Autodesk Inventor part; units mm, degrees
ref_plane "YZ Plane" through (0, 0, 0) normal (1, 0, 0) x (0, 1, 0)
ref_plane "XZ Plane" through (0, 0, 0) normal (0, 1, 0) x (-1, 0, 0)
ref_plane "XY Plane" through (0, 0, 0) normal (0, 0, 1) x (1, 0, 0)
sketch "Sketch1" plane through (0, 0, 0) normal (0, 1, 0) x (-1, 0, 0)
  circle A0 centre (0, 0) radius 11.05
  line L0 (21.25, 17.25) -> (21.25, -17.25)
  line L1 (21.25, -17.25) -> (17.25, -21.25)
  line L2 (17.25, -21.25) -> (-17.25, -21.25)
  line L3 (-17.25, -21.25) -> (-21.25, -17.25)
  line L4 (-21.25, -17.25) -> (-21.25, 17.25)
  line L5 (-21.25, 17.25) -> (-17.25, 21.25)
  line L6 (-17.25, 21.25) -> (17.25, 21.25)
  line L7 (17.25, 21.25) -> (21.25, 17.25)
  line L8 (21.25, 0) -> (-21.25, 0) construction
  line L9 (0, 21.25) -> (0, -21.25) construction
  circle A1 centre (15.3506, -15.3506) radius 1.55
  line L10 (15.3506, -15.3506) -> (0, 0) construction
  circle A2 centre (15.3506, 15.3506) radius 1.55
  circle A3 centre (-15.3506, 15.3506) radius 1.55
  circle A4 centre (-15.3506, -15.3506) radius 1.55
  point P0 (0, 0)
  dimension "d0" = 22.1
  dimension "d1" = 135
  dimension "d2" = 42.5
  dimension "d3" = 5.6569
  dimension "d25" = 3.1
  dimension "d26" = 21.709
  dimension "d27" = 45
  dimension "d30" = 360
extrude "Extrusion1" add sketch "Sketch1" along normal blind 6
sketch "Sketch6" plane through (0, 0, 0) normal (0, -1, 0) x (1, 0, 0)
  line L0 (27.25, -23.25) -> (27.25, 23.25)
  line L1 (27.25, 23.25) -> (23.25, 27.25)
  line L2 (23.25, 27.25) -> (-23.25, 27.25)
  line L3 (-23.25, 27.25) -> (-27.25, 23.25)
  line L4 (-27.25, 23.25) -> (-27.25, -23.25)
  line L5 (-27.25, -23.25) -> (-23.25, -27.25)
  line L6 (-23.25, -27.25) -> (23.25, -27.25)
  line L7 (23.25, -27.25) -> (27.25, -23.25)
  line L8 (25.25, -25.25) -> (-25.25, 25.25) construction
  line L9 (-17.25, 21.25) -> (17.25, 21.25) construction
  line L10 (23.25, 27.25) -> (17.25, 21.25) construction
  line L11 (27.25, 23.25) -> (21.25, 17.25) construction
  line L12 (21.25, -17.25) -> (17.25, -21.25)
  line L13 (21.25, 17.25) -> (21.25, -17.25)
  line L14 (21.25, -17.25) -> (21.25, 17.25)
  line L15 (17.25, 21.25) -> (21.25, 17.25)
  line L16 (21.25, 17.25) -> (17.25, 21.25)
  line L17 (17.25, 21.25) -> (-17.25, 21.25)
  line L18 (-21.25, 17.25) -> (-17.25, 21.25)
  line L19 (-21.25, 17.25) -> (-17.25, 21.25)
  line L20 (17.25, 21.25) -> (21.25, 17.25)
  line L21 (-21.25, -17.25) -> (-21.25, 17.25)
  line L22 (-21.25, 17.25) -> (-21.25, -17.25)
  line L23 (-21.25, -17.25) -> (-17.25, -21.25)
  line L24 (-17.25, -21.25) -> (17.25, -21.25)
  line L25 (17.25, -21.25) -> (21.25, -17.25)
  point P0 (0, 0)
  point P1 (0, 0)
  dimension "d32" = 135
  dimension "d33" = 135
  dimension "d34" = 46.5
extrude "Extrusion5" add sketch "Sketch6" against normal blind 41
sketch "Sketch8" plane through (0, 41, 0) normal (0, 1, 0) x (1, 0, 0)
  line L0 (27.25, -23.25) -> (27.25, 23.25)
  line L1 (21.25, -17.25) -> (21.25, 17.25)
  line L2 (27.25, 23.25) -> (21.25, 17.25)
  line L3 (17.25, -21.25) -> (21.25, -17.25)
  line L4 (21.25, 17.25) -> (21.25, -17.25)
  line L5 (21.25, -17.25) -> (27.25, -23.25)
  line L6 (27.25, -23.25) -> (27.25, 23.25)
  point P0 (0, 0)
  point P1 (27.25, -23.25)
extrude "Extrusion6" cut sketch "Sketch8" against normal blind 35
sketch "Sketch9" plane through (0, 6, 0) normal (0, 1, 0) x (1, 0, 0)
  line L0 (23.25, 27.25) -> (-23.25, 27.25)
  line L1 (17.25, 21.25) -> (21.25, 17.25)
  line L2 (23.25, 27.25) -> (17.25, 21.25)
  line L3 (-21.25, 17.25) -> (-17.25, 21.25)
  line L4 (17.25, 21.25) -> (-17.25, 21.25)
  line L5 (-17.25, 21.25) -> (-23.25, 27.25)
  line L6 (-23.25, 27.25) -> (23.25, 27.25)
  line L7 (-17.25, -21.25) -> (17.25, -21.25)
  line L8 (23.25, -27.25) -> (-23.25, -27.25)
  line L9 (17.25, -21.25) -> (23.25, -27.25)
  line L10 (23.25, -27.25) -> (-23.25, -27.25)
  line L11 (-23.25, -27.25) -> (-17.25, -21.25)
  line L12 (-17.25, -21.25) -> (17.25, -21.25)
  point P0 (0, 0)
  point P1 (-23.25, 27.25)
extrude "Extrusion7" cut sketch "Sketch9" along normal blind 29
sketch "Sketch10" plane through (-21.25, 6, -17.25) normal (1, 0, 0) x (0, 0, -1)
  line L0 (6, 0) -> (-40.5, 0) construction
  line L1 (-17.25, 0) -> (-17.25, 35) construction
  line L2 (-34.5, 35) -> (0, 35) construction
  line L3 (0, 0) -> (0, 35) construction
  line L4 (0, 17.5) -> (-34.5, 17.5) construction
  line L5 (-34.5, 0) -> (-34.5, 35) construction
  line L6 (-32.5, 2) -> (-2, 2)
  line L7 (-2, 2) -> (-2, 33)
  line L8 (-2, 33) -> (-32.5, 33)
  line L9 (-32.5, 33) -> (-32.5, 2)
  line L10 (-17.25, 2) -> (-17.25, 33) construction
  line L11 (-32.5, 17.5) -> (-2, 17.5) construction
  point P0 (-17.25, -6)
  point P1 (-17.25, 17.5)
  dimension "d41" = 2
  dimension "d42" = 2
extrude "Extrusion8" cut sketch "Sketch10" against normal blind 2
sketch "Sketch11" plane through (-23.25, 6, -17.25) normal (1, 0, 0) x (0, 0, -1)
  line L0 (-7.2, 7.5) -> (-27.3, 7.5) construction
  line L1 (-27.3, 7.5) -> (-27.3, 27.5) construction
  line L2 (-27.3, 27.5) -> (-7.2, 27.5) construction
  line L3 (-7.2, 27.5) -> (-7.2, 7.5) construction
  line L4 (-2, 33) -> (-2, 2) construction
  line L5 (-32.5, 2) -> (-32.5, 33) construction
  line L6 (-2, 2) -> (-32.5, 33) construction
  line L7 (-32.5, 33) -> (-2, 33) construction
  line L8 (-32.5, 2) -> (-2, 33) construction
  line L9 (-7.2, 7.5) -> (-27.3, 27.5) construction
  line L10 (-27.3, 7.5) -> (-7.2, 27.5) construction
  point P0 (-17.25, -6)
  point P1 (-17.25, 17.5)
  dimension "d45" = 20.1
  dimension "d46" = 20
hole "Hole2" at (-23.25, 13.5, -10.05) at (-23.25, 13.5, 10.05) at (-23.25, 33.5, -10.05) at (-23.25, 33.5, 10.05) direction (-1, 0, 0) diameter 3 depth 4
equation "\"d0\" = shaft_hole_diameter"
equation "\"d4\" = mount_face_thickness"
equation "\"d34\" = mount_width"
equation "\"d35\" = mount_length"
equation "\"d37\" = mount_length - mount_face_thickness"
equation "\"d39\" = mount_length - 2 * mount_face_thickness"
equation "\"d45\" = screw_x"
equation "\"d46\" = screw_y"
equation "\"d47\" = screw_diameter"
equation "\"shaft_hole_diameter\" = 22.1"
equation "\"mount_width\" = 46.5"
equation "\"mount_slant_length\" = 5"
equation "\"mount_face_thickness\" = 6"
equation "\"mount_length\" = 41"
equation "\"screw_x\" = 20.1"
equation "\"screw_y\" = 20"
equation "\"screw_diameter\" = 3"
properties part number "table_motor_mount"
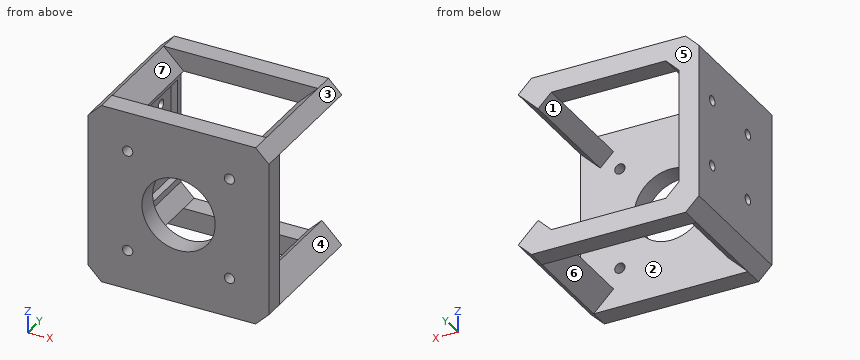
The model under review builds one solid part; all positions refer to its coordinate system, in mm. Face numbers are marked on the shaded views. A direction names the side the tool comes from. Round coordinates to 2 decimals unless told otherwise and drop trailing zeros. Loops run counter-clockwise (first coordinate to the right, second up) from the corner with the lowest first, then second, coordinate; pieces in that order, holes last. Notation, with made-up numbers: M 44.5,81 L 62.5,81 A14 cw 62.5,87 Z; hole C -6.5,-30.75 d5. An arc over 180 degrees is marked long. Answer as CSV lines item,"result". Start each with the question number.
Item 1: Insertion check: P1, Ø3, axis at x = -15.35, z = 15.35, coming from the +Y side; P2, Ø4, axis at x = 15.35, z = -15.35, coming from the +Y side; P3, Ø0.6, axis at x = -22, y = 23.5, coming from the +Z side; P4, Ø2, axis at x = -22, y = 19, coming from the -Z side. Each pin has a flat end and moves straight along its axis. Give the tip position at first contact, or say it passes through.
Item 2: Consider section A-A (z = 0). Write out the cut boundary in (x, y), then the cut area to 3 significant figures.
Item 3: Mouldability with a two-part tool opening along Y and no side actions: class the marked faces 4, 5, 6 and 7 as released by +Y, released by -Y, zero draft, split by the parting line, or undercut.
Item 4: Consider section B-B (y = 33.5). Write out the cut boundary in (x, z), then the cut area to 3 significant figures.
Item 5: Consider section D-D (x = -18.5). Write out the cut boundary in (y, z).
Item 6: Wall thickness on line 1 (Y direction, x = -24, z = -10); line 2 (Z direction, x = 0, y = 1); line 3 (Z direction, x = -25.4, y = 33.5): over which ranges is each line inside the solid? List them lowest first. Write a range as [from, to].
Item 7: Consider section C-C (x = 0). Write out the cut boundary in (y, z).
Item 8: For the marked faces 1, 2 and 3, list the 3-axis set-ups (+Z, -Z, +X, -X, +Y, -Y) from which the entire face can be reached by the end or side of a thin tool; tool diameter is ignored.
Answer:
1,P1,"passes through"
1,P2,"stops at y = 6"
1,P3,"stops at z = 26.3"
1,P4,"stops at z = -27"
2,outline,"M -27.25,0 L -11.05,0 L -11.05,6 L -21.25,6 L -21.25,8 L -23.25,8 L -23.25,39 L -21.25,39 L -21.25,41 L -27.25,41 Z; M 11.05,0 L 27.25,0 L 27.25,6 L 11.05,6 Z"
2,area,"342 mm^2"
3,face 4,"zero draft"
3,face 5,"released by +Y"
3,face 6,"undercut"
3,face 7,"undercut"
4,outline,"M -27.25,-23.25 L -23.25,-27.25 L -17.25,-21.25 L -21.25,-17.25 L -21.25,-15.25 L -23.25,-15.25 L -23.25,-11.55 L -27.25,-11.55 Z; M -27.25,-8.55 L -23.25,-8.55 L -23.25,8.55 L -27.25,8.55 Z; M -27.25,11.55 L -23.25,11.55 L -23.25,15.25 L -21.25,15.25 L -21.25,17.25 L -17.25,21.25 L -23.25,27.25 L -27.25,23.25 Z; M 17.25,-21.25 L 23.25,-27.25 L 27.25,-23.25 L 21.25,-17.25 Z; M 17.25,21.25 L 21.25,17.25 L 27.25,23.25 L 23.25,27.25 Z"
4,area,"350 mm^2"
5,outline,"M 0,-27.25 L 6,-27.25 L 6,-22.5 L 35,-22.5 L 35,-27.25 L 41,-27.25 L 41,-20 L 6,-20 L 6,20 L 41,20 L 41,27.25 L 35,27.25 L 35,22.5 L 6,22.5 L 6,27.25 L 0,27.25 Z"
6,line 1,"y = [0, 12], [15, 32], [35, 41]"
6,line 2,"z = [-27.25, -11.05], [11.05, 27.25]"
6,line 3,"z = [-25.1, -11.55], [-8.55, 8.55], [11.55, 25.1]"
7,outline,"M 0,-27.25 L 6,-27.25 L 6,-11.05 L 0,-11.05 Z; M 0,11.05 L 6,11.05 L 6,27.25 L 0,27.25 Z; M 35,-27.25 L 41,-27.25 L 41,-21.25 L 35,-21.25 Z; M 35,21.25 L 41,21.25 L 41,27.25 L 35,27.25 Z"
8,face 1,"+Y"
8,face 2,"none"
8,face 3,"+Z, +X, +Y, -Y"
